from build123d import *

# Parameters (mm, degrees)
BOSS_EXTRUDE1_DEPTH = 5
FILLET1_R           = 5
FILLET2_R           = 5
FILLET3_R           = 2
SKETCH2_R           = 1.7
CUT_EXTRUDE1_DEPTH  = 147


with BuildPart() as part:
    # Sketch1 → Boss-Extrude1 (new, symmetric)
    with BuildSketch(Plane.XY):
        with BuildLine():
            ThreePointArc((-63, -10), (-60.071067812, -2.928932188), (-53, 0))
            Line((-53, 0), (0, 0))
            Line((0, 0), (0, 10))
            Line((0, 10), (-71, 10))
            Line((-71, 10), (-71, 0))
            Line((-71, 0), (-71, -28))
            Line((-71, -28), (-63, -28))
            Line((-63, -28), (-63, -10))
        make_face()
        with BuildLine():
            Line((0, 10), (0, 0))
            Line((0, 0), (53, 0))
            ThreePointArc((53, 0), (60.071067812, -2.928932188), (63, -10))
            Line((63, -10), (63, -28))
            Line((63, -28), (71, -28))
            Line((71, -28), (71, 0))
            Line((71, 0), (71, 10))
            Line((71, 10), (0, 10))
        make_face()
    extrude(amount=BOSS_EXTRUDE1_DEPTH, both=True)

    # Fillet1
    fillet1_edges = [part.edges().sort_by_distance(p)[0] for p in [
        (-67, -28, -5),
        (-67, -28, 5),
        (67, -28, -5),
        (67, -28, 5),
    ]]
    fillet(fillet1_edges, radius=FILLET1_R - 0.0001)  # a hair under: the kernel refuses the full size

    # Fillet2
    fillet2_edges = [part.edges().sort_by_distance(p)[0] for p in [
        (0, 10, -5),
        (-71, 10, 0),
        (71, 10, 0),
        (0, 10, 5),
    ]]
    fillet(fillet2_edges, radius=FILLET2_R - 0.0001)  # a hair under: the kernel refuses the full size

    # Fillet3
    fillet3_edges = [part.edges().sort_by_distance(p)[0] for p in [
        (0, 0, 5),
        (-63, -16.50005, -5),
        (63, -16.50005, -5),
        (60.071067812, -2.928932188, -5),
        (60.071067812, -2.928932188, 5),
        (0, 0, -5),
        (-60.071067812, -2.928932188, -5),
        (63, -16.50005, 5),
        (-63, -26.535563195, 3.535563195),
        (-63, -26.535563195, -3.535563195),
        (63, -26.535563195, 3.535563195),
        (63, -26.535563195, -3.535563195),
        (-60.071067812, -2.928932188, 5),
        (-63, -16.50005, 5),
    ]]
    fillet(fillet3_edges, radius=FILLET3_R)

    # Sketch2 → Cut-Extrude1 (cut)
    with BuildSketch(Plane(origin=(71, 0, 0), x_dir=(0, 0, -1), z_dir=(1, 0, 0))):
        with Locations((0, -20.652619003)):
            Circle(SKETCH2_R)
    extrude(amount=-CUT_EXTRUDE1_DEPTH, mode=Mode.SUBTRACT)


solid = part.part
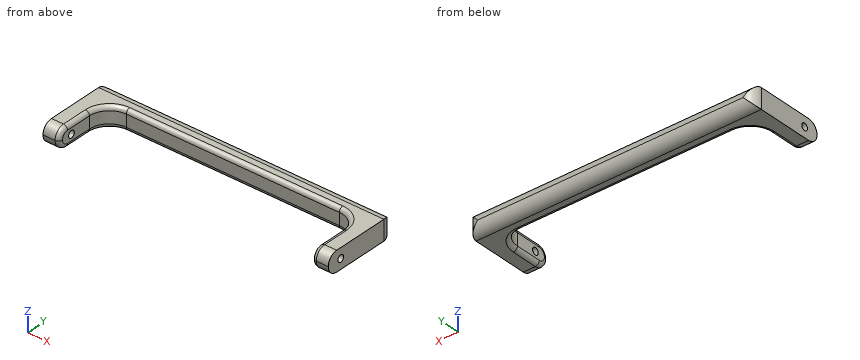
Verification items for the finished model (mm, model axes). Give positions to 0.01 mm unless a question says otherwise; leave off trailing zeros. Order: outer loops, then holes, each group sorted by start corner. A loop starts at its lowest first (then second) coordinate and runs counter-clockwise, first axis right, second up. Notation, with made-up numbers: M 2,81.25 L 9,81.25 A27 ccw 9,110.25 Z; hole C 34,3 d11. An arc over 180 degrees is marked long. Use one line per item in the form item = value. Start each with the question number.
Q1. Section check A-A (y = -13). Enter the section's corners in (x, z), then the cut area to 3 significant figures.
Q2. Scan lines: line 1 along Y through (x, z) = (66, 0); line 2 along X through (y, z) = (-9.5, -1.5); line 3 along Y through (x, z) = (3.5, 0). Record each from-to range of solid material in increasing order. Write a range as [from, to].
Q3. Go/stop test with flat-tipped pins: pin 1 Ø5 at (x, z) = (-7, -1) entering from -Y; pin 2 Ø10 at (x, y) = (-12, -4) entering from -Z; pin 3 Ø1 at (x, z) = (-16.5, 1) entering from +Y. Record where each tip stops, or that it passes through.
Evaluation:
q1.outline = M -71,-5 L -65,-5 A2 ccw -63,-3 L -63,3 A2 ccw -65,5 L -71,5 Z; M 63,-3 A2 ccw 65,-5 L 71,-5 L 71,5 L 65,5 A2 ccw 63,3 Z
q1.area = 157 mm2
q2.line_1 = [-28, -22.35], [-18.95, 10]
q2.line_2 = [-71, -62.99], [62.99, 71]
q2.line_3 = [0, 10]
q3.pin_1 = 0
q3.pin_2 = -4.73
q3.pin_3 = 9.97
